```python
from build123d import *

# Parameters (mm, degrees)
CHAMFER2_SIZE     = 3.81
HOLE1_D           = 6
HOLE1_DEPTH       = 3
CIRPATTERN1_COUNT = 10
CHAMFER3_SIZE     = 2.54


with BuildPart() as part:
    # Sketch1 → Revolve1 (revolve)
    with BuildSketch(Plane.XY, mode=Mode.PRIVATE) as revolve1_sk:
        Polygon((19.939, 0), (43.84802, 0), (43.84802, 15.24), (31.75, 15.24), (31.75, 6.35), (23.749, 6.35), (23.749, 14.33322), (19.939, 14.33322), align=None)
    revolve(revolve1_sk.sketch.rotate(Axis((0, 0, 0), (0, 1, 0)), 90), axis=Axis((0, 0, 0), (0, 1, 0)))

    # Chamfer2
    chamfer2_edges = [part.edges().sort_by_distance(p)[0] for p in [
        (0, 14.33322, 23.749),
    ]]
    chamfer(chamfer2_edges, length=CHAMFER2_SIZE - 0.0001)  # a hair under: the kernel refuses the full size

    # Hole1
    with Locations(Plane(origin=(0, 15.24, 0), x_dir=(1, 0, 0), z_dir=(0, 1, 0))):
        with Locations((38.1, 0)):
            hole1 = Hole(HOLE1_D / 2, depth=HOLE1_DEPTH)

    # Sketch5 → M4x0.7 Tapped Hole1 (revolve, cut)
    with BuildSketch(Plane(origin=(38.1, 12.24, 0), x_dir=(0, 0, 1), z_dir=(1, 0, 0))):
        Polygon((0, 0), (0, 8.991429421), (1.65, 8.0000094), (1.65, 0), align=None)
    m4x0_7_tapped_hole1 = revolve(axis=Axis((38.1, 18.59, 0), (0, -1, 0)), mode=Mode.SUBTRACT)

    # CirPattern1: Hole1, M4x0.7 Tapped Hole1 ×10 about axis
    cirpattern1_axis = Axis((0, 0, 0), (0, 1, 0))
    add([hole1.rotate(cirpattern1_axis, i * 360 / CIRPATTERN1_COUNT) for i in range(1, CIRPATTERN1_COUNT)], mode=Mode.SUBTRACT)
    add([m4x0_7_tapped_hole1.rotate(cirpattern1_axis, i * 360 / CIRPATTERN1_COUNT) for i in range(1, CIRPATTERN1_COUNT)], mode=Mode.SUBTRACT)

    # Chamfer3
    chamfer3_edges = [part.edges().sort_by_distance(p)[0] for p in [
        (0, 0, 43.84802),
    ]]
    chamfer(chamfer3_edges, length=CHAMFER3_SIZE)


solid = part.part
```
The listing builds one solid part. Answer for the finished solid, in the listing's coordinates (mm). A direction names the side the tool comes from. Give positions to 0.01 mm unless a question says otherwise; leave off trailing zeros. Use one line per item in the form item = value.
1) A tool of negligible diameter and unlimited length cuts with its end or side. For faces 1 (the conical face through (36.79, 0.16, -19.13)), 2 (the cylindrical face through (33.071, 13.719, -20.408)), from which of +Z, -Z, +X, -X, +Y, -Y can it reach the whole face along a straight path? Write none if from no direction.
Result:
face_1 = -Y
face_2 = +Y
2) Straight lines are drawn through the part: probe 1 along X at (y, z) = (14, 13); probe 2 along X at (y, z) = (14, 1); probe 3 along Z at (x, y) = (29.5, 14). For each, find the intervals that lie inside material, in ascending order.
Result:
probe_1 = -41.88 to -28.97, -15.56 to -15.12, 15.12 to 15.56, 28.97 to 41.88
probe_2 = -43.84 to -40.93, -35.27 to -31.73, -20.25 to -19.91, 19.91 to 20.25, 31.73 to 35.27, 40.93 to 43.84
probe_3 = -32.44 to -25.09, -19.7 to -11.74, 11.74 to 19.7, 25.09 to 32.44
3) Each of these flat-tipped pins is pushed along its axis until it touches: P1, Ø12, axis at x = -12, z = -11.5, coming from the +Y side; P2, Ø5, axis at x = 30.82, z = -22.39, coming from the +Y side; P3, Ø2, axis at y = 5.5, z = 18, coming from the -X side. Where does it stop, or does it pass through?
Result:
P1 = 14.33
P2 = 12.24
P3 = -40.42
4) Section A-A on y = 8.75 is taken. Count the separate pieces of the cut face and the enclosed holes in it, plus the area to 3 significant figures.
Result:
separate_pieces = 2
enclosed_holes = 12
area = 3,310 mm²
5) For a pull along X with two mould halves and no side action, classify faces 3 (the conical face through (37.82, 3.42, -0.04)), 4 (the flat face through (18, 0, -10)), 5 (the cylindrical face through (26.681, 8.979, 34.796)) as +X half, -X half, draft (parallel to the pull), parting line (faces both ways), or undercut.
Result:
face_3 = undercut
face_4 = draft
face_5 = parting line
